The model under review builds one solid part; all positions refer to its coordinate system, in mm. Face numbers are marked on the shaded views. A direction names the side the tool comes from. Coordinates: 2 decimals unless noted, no trailing zeros. Loops run counter-clockwise (first coordinate to the right, second up) from the corner with the lowest first, then second, coordinate; pieces in that order, holes last. Notation, with made-up numbers: (20, 30.25) - (36, 30.25) arc R15 ccw to (36, 52.25) - close; hole circle Ø8 at (29, -6.5). An arc over 180 degrees is marked (long way). Use a Markdown table: item, result. Add a question column.
1) Add section C-C, the plane x = 26.5. Give the boundary of the cut face in (y, z), and give its area (3 significant figures).
2) For the marked faces 4, 5 and 6, list the 3-axis set-ups (+Z, -Z, +X, -X, +Y, -Y) from which the entire face can be reached by the end or side of a thin tool; tool diameter is ignored.
3) Add section D-D, the plane x = 10. Give the boundary of the cut face in (y, z), and give its area (3 significant figures).
4) The part is to be moulded in two halves that separate along Y. For the marked faces 1, 2 and 3, say which applies: pulls with the +Y half, pulls with the -Y half, needs draft (parallel to the pull), parting line crosses it, or undercut.
5) To check wall thickness, follow L1, parallel to Z at x = 35.5, y = 0; L2, parallel to Y at x = 16.5, z = -4; L3, parallel to Y at x = 39.5, z = 5. State the ranges of each line that lie inside material, in increasing order. Write a range as [from, to].
6) Add section A-A, the plane y = 0. Give the boundary of the cut face in (x, z).
7) Clearance check with flat-ended pins moving along their axes: pin 1 (5 mm diameter, centred on x = 31.5, y = -8.5, fed in from +Z); pin 2 (5 mm diameter, centred on x = 11.5, z = 13, fed in from -Y); pin 3 (2 mm diameter, centred on y = -39.5, z = -22.5, fed in from +X). State where each tip first meets the part, or that it passes through.
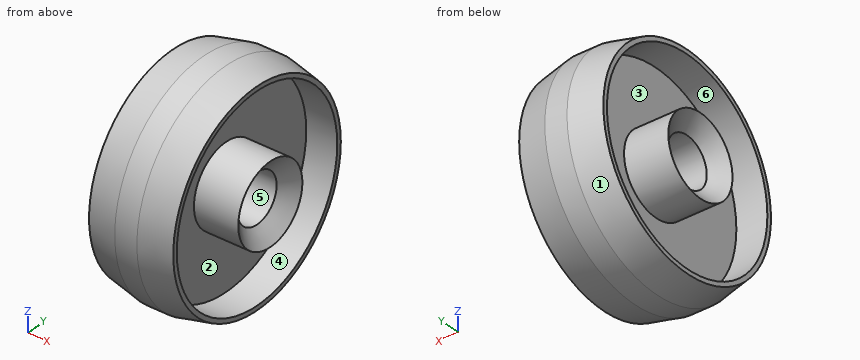
Autodesk Inventor part; units mm, degrees
ref_plane "YZ Plane" through (0, 0, 0) normal (1, 0, 0) x (0, 1, 0)
ref_plane "XZ Plane" through (0, 0, 0) normal (0, 1, 0) x (-1, 0, 0)
ref_plane "XY Plane" through (0, 0, 0) normal (0, 0, 1) x (1, 0, 0)
sketch "Sketch1" plane through (0, 0, 0) normal (0, 0, 1) x (1, 0, 0)
  line L0 (0, 0) -> (50, 0)
  line L1 (6, 11) -> (44, 11)
  line L2 (20, 50) -> (30, 50)
  line L3 (20, 18) -> (20, 45)
  line L4 (30, 18) -> (30, 45)
  line L5 (0, 18) -> (20, 18)
  line L6 (30, 18) -> (50, 18)
  line L7 (44, 45) -> (44, 47)
  line L8 (6, 45) -> (6, 47)
  line L9 (44, 47) -> (30, 50)
  line L10 (20, 50) -> (6, 47)
  line L11 (6, 45) -> (20, 45)
  line L12 (30, 45) -> (44, 45)
  line L13 (50, 18) -> (44, 11)
  line L14 (6, 11) -> (0, 18)
  dimension "d0" = 50
  dimension "d2" = 38
  dimension "d3" = 11
  dimension "d4" = 39
  dimension "d8" = 10
  dimension "d9" = 20
  dimension "d12" = 2
  dimension "d13" = 2
  dimension "d14" = 18
  dimension "d15" = 26.2486
  dimension "d16" = 11.7142
  dimension "d17" = 18
  dimension "d18" = 45
revolve "Revolution1" add sketch "Sketch1" angle 360 about axis through (0, 0, 0) along (1, 0, 0)
properties part number "wheel" material "Iron, Malleable"
From the geometry:
| question | item | result |
|---|---|---|
| 1 | outline | circle Ø100 at (0, 0); hole circle Ø22 at (0, 0) |
| 1 | area | 7,470 mm^2 |
| 2 | face 4 | +X |
| 2 | face 5 | +X, -X |
| 2 | face 6 | -X |
| 3 | outline | circle Ø95.71 at (0, 0); circle Ø36 at (0, 0); hole circle Ø90 at (0, 0); hole circle Ø22 at (0, 0) |
| 3 | area | 1,470 mm^2 |
| 4 | face 1 | parting line crosses it |
| 4 | face 2 | undercut |
| 4 | face 3 | undercut |
| 5 | L1 | z = [-48.82, -45], [-18, -11], [11, 18], [45, 48.82] |
| 5 | L2 | y = [-49.09, -44.82], [-17.55, -10.25], [10.25, 17.55], [44.82, 49.09] |
| 5 | L3 | y = [-47.7, -44.72], [-17.29, -9.8], [9.8, 17.29], [44.72, 47.7] |
| 6 | outline | (0, -18) - (20, -18) - (20, -45) - (6, -45) - (6, -47) - (20, -50) - (30, -50) - (44, -47) - (44, -45) - (30, -45) - (30, -18) - (50, -18) - (44, -11) - (6, -11) - close; (0, 18) - (6, 11) - (44, 11) - (50, 18) - (30, 18) - (30, 45) - (44, 45) - (44, 47) - (30, 50) - (20, 50) - (6, 47) - (6, 45) - (20, 45) - (20, 18) - close |
| 7 | pin 1 | stops at z = 49.58 |
| 7 | pin 2 | stops at y = -47.24 |
| 7 | pin 3 | stops at x = 44 |
